from build123d import *

# Parameters (mm, degrees)
CROQUIS1_R              = 7.5
SALIENTE_EXTRUIR2_DEPTH = 30
REDONDEO1_R             = 25
CROQUIS2_R              = 7.5
SALIENTE_EXTRUIR3_DEPTH = 50
REDONDEO2_R             = 5
REDONDEO4_R             = 15


# Some blends are built 0.0001 mm under size
with BuildPart() as part:
    # Croquis1 → Saliente-Extruir2 (new body)
    with BuildSketch(Plane.XY):
        Polygon((12.5, 0), (12.5, 60), (37.5, 60), (37.5, 0), (50, 0), (50, 350), (0, 350), (0, 0), align=None)
        with Locations((25, 325)):
            Circle(CROQUIS1_R, mode=Mode.SUBTRACT)
    extrude(amount=SALIENTE_EXTRUIR2_DEPTH)

    # Redondeo1
    redondeo1_edges = [part.edges().sort_by_distance(p)[0] for p in [
        (0, 350, 15),
        (50, 350, 15),
    ]]
    fillet(redondeo1_edges, radius=REDONDEO1_R - 0.0001)  # a hair under: the kernel refuses the full size

    # Croquis2 → Saliente-Extruir3 (add)
    with BuildSketch(Plane.ZY):
        with Locations((15, 25)):
            Circle(CROQUIS2_R)
    extrude(amount=-SALIENTE_EXTRUIR3_DEPTH)

    # Redondeo2
    redondeo2_edges = [part.edges().sort_by_distance(p)[0] for p in [
        (12.5, 30, 30),
        (25, 60, 30),
        (50, 0, 15),
        (37.5, 0, 15),
        (12.5, 0, 15),
        (0, 0, 15),
        (37.5, 30, 30),
        (50, 162.50005, 30),
        (0, 162.50005, 0),
        (0, 162.50005, 30),
        (42.677698819, 342.677698819, 0),
        (7.322301181, 342.677698819, 0),
        (42.677698819, 342.677698819, 30),
        (7.322301181, 342.677698819, 30),
        (50, 162.50005, 0),
        (37.5, 30, 0),
        (25, 60, 0),
        (12.5, 30, 0),
    ]]
    fillet(redondeo2_edges, radius=REDONDEO2_R)

    # Redondeo4
    # the kernel refuses this fillet: 15 mm, written as the material it takes off along each edge
    with BuildSketch(Plane(origin=(50, 15, 15), x_dir=(0, -1, 0), z_dir=(0, 0, 1))) as redondeo4_piece_1:
        with BuildLine():
            CenterArc((10, -5), 5, 0, 90)
            Line((15, -5), (15, 0))
            Line((15, 0), (10, 0))
        make_face()
    revolve(axis=Axis((50, 15, 15), (1, 0, 0)), revolution_arc=90, mode=Mode.SUBTRACT)
    with BuildSketch(Plane(origin=(37.5, 15, 15), x_dir=(0, 0, -1), z_dir=(0, 1, 0))) as redondeo4_piece_2:
        with BuildLine():
            CenterArc((10, -5), 5, 0, 90)
            Line((15, -5), (15, 0))
            Line((15, 0), (10, 0))
        make_face()
    revolve(axis=Axis((37.5, 15, 15), (-1, 0, 0)), revolution_arc=90, mode=Mode.SUBTRACT)
    with BuildSketch(Plane(origin=(12.5, 15, 15), x_dir=(0, -1, 0), z_dir=(0, 0, 1))) as redondeo4_piece_3:
        with BuildLine():
            CenterArc((10, -5), 5, 0, 90)
            Line((15, -5), (15, 0))
            Line((15, 0), (10, 0))
        make_face()
    revolve(axis=Axis((12.5, 15, 15), (1, 0, 0)), revolution_arc=90, mode=Mode.SUBTRACT)
    with BuildSketch(Plane(origin=(0, 15, 15), x_dir=(0, 0, -1), z_dir=(0, 1, 0))) as redondeo4_piece_4:
        with BuildLine():
            CenterArc((10, -5), 5, 0, 90)
            Line((15, -5), (15, 0))
            Line((15, 0), (10, 0))
        make_face()
    revolve(axis=Axis((0, 15, 15), (-1, 0, 0)), revolution_arc=90, mode=Mode.SUBTRACT)
    with BuildSketch(Plane(origin=(12.5, 15, 15), x_dir=(0, 0, 1), z_dir=(0, 1, 0))) as redondeo4_piece_5:
        with BuildLine():
            CenterArc((10, -5), 5, 0, 90)
            Line((15, -5), (15, 0))
            Line((15, 0), (10, 0))
        make_face()
    revolve(axis=Axis((12.5, 15, 15), (1, 0, 0)), revolution_arc=90, mode=Mode.SUBTRACT)
    with BuildSketch(Plane(origin=(0, 15, 15), x_dir=(0, -1, 0), z_dir=(0, 0, -1))) as redondeo4_piece_6:
        with BuildLine():
            CenterArc((10, -5), 5, 0, 90)
            Line((15, -5), (15, 0))
            Line((15, 0), (10, 0))
        make_face()
    revolve(axis=Axis((0, 15, 15), (-1, 0, 0)), revolution_arc=90, mode=Mode.SUBTRACT)
    with BuildSketch(Plane(origin=(50, 15, 15), x_dir=(0, 0, 1), z_dir=(0, 1, 0))) as redondeo4_piece_7:
        with BuildLine():
            CenterArc((10, -5), 5, 0, 90)
            Line((15, -5), (15, 0))
            Line((15, 0), (10, 0))
        make_face()
    revolve(axis=Axis((50, 15, 15), (1, 0, 0)), revolution_arc=90, mode=Mode.SUBTRACT)
    with BuildSketch(Plane(origin=(37.5, 15, 15), x_dir=(0, -1, 0), z_dir=(0, 0, -1))) as redondeo4_piece_8:
        with BuildLine():
            CenterArc((10, -5), 5, 0, 90)
            Line((15, -5), (15, 0))
            Line((15, 0), (10, 0))
        make_face()
    revolve(axis=Axis((37.5, 15, 15), (-1, 0, 0)), revolution_arc=90, mode=Mode.SUBTRACT)
    with BuildSketch(Plane(origin=(37.5, 0, 30), x_dir=(0, 1, 0), z_dir=(1, 0, 0)), Plane(origin=(0, 0, 30), x_dir=(0, 1, 0), z_dir=(1, 0, 0))) as redondeo4_piece_9:
        with BuildLine():
            CenterArc((REDONDEO4_R, -REDONDEO4_R), REDONDEO4_R, 90, 90)
            Line((0, -REDONDEO4_R), (0, 0))
            Line((0, 0), (REDONDEO4_R, 0))
        make_face()
    extrude(amount=12.5, mode=Mode.SUBTRACT)
    with BuildSketch(Plane(origin=(0, 0, 0), x_dir=(0, 1, 0), z_dir=(1, 0, 0)), Plane(origin=(37.5, 0, 0), x_dir=(0, 1, 0), z_dir=(1, 0, 0))) as redondeo4_piece_10:
        with BuildLine():
            CenterArc((REDONDEO4_R, REDONDEO4_R), REDONDEO4_R, 180, 90)
            Line((0, REDONDEO4_R), (0, 0))
            Line((0, 0), (REDONDEO4_R, 0))
        make_face()
    extrude(amount=12.5, mode=Mode.SUBTRACT)


solid = part.part
Model file for the job. Use its own axes, mm. A direction names the side the tool comes from. Round coordinates to 2 decimals unless told otherwise and drop trailing zeros. Loops run counter-clockwise (first coordinate to the right, second up) from the corner with the lowest first, then second, coordinate; pieces in that order, holes last. Notation, with made-up numbers: (-20.75, 64) - (14.25, 64) arc R30 cw to (14.25, 100) - close; hole circle Ø1 at (-2.5, 47.25). An arc over 180 degrees is marked (long way). Write each question's results on one line, items separated by ' | '.
(1) 3-axis set-ups, long thin cutter, end or side, ignore diameter. For faces 4 (the flat face through (25, 60, 15)), 5 (the cylindrical face through (24.825, 32.436, 14.024)), 6 (the flat face through (50, 163, 15)): which of +Z, -Z, +X, -X, +Y, -Y reach the whole face in a straight line?
Answer below:
face 4: +Z, -Z | face 5: none | face 6: +Z, -Z, +X, +Y, -Y
(2) Saw through at A-A, the plane z = 15. Count the separate pieces of the cut face and the enclosed holes in it, then the cut area to 3 significant figures.
Answer below:
separate pieces: 1 | enclosed holes: 2 | area: 15,900 mm^2
(3) Wall check: L1, parallel to Y at x = 24.5, z = 15.25 (3 decimals); L2, parallel to Y at x = 25, z = 11; L3, parallel to X at y = 325, z = 19.25. Give the ranges that are in metal, low to high.
Answer below:
L1: y = 17.504 to 32.496, 60 to 317.517, 332.483 to 349.995 | L2: y = 18.66 to 31.34, 60 to 317.5, 332.5 to 350 | L3: x = 0 to 17.5, 32.5 to 50
(4) Pin check, flat tips, straight feed: pin 1 (10 mm diameter, centred on x = 30.5, z = 18, fed in from -Y); pin 2 (5 mm diameter, centred on x = 31, z = 21, fed in from -Y); pin 3 (1.5 mm diameter, centred on x = 26.5, z = 15, fed in from +Y). Stop position of each tip, or through.
Answer below:
pin 1: stops at y = 17.5 | pin 2: stops at y = 18.37 | pin 3: stops at y = 349.99
(5) Saw through at B-B, the plane y = 25. List the corners of the cut face in (x, z), then the cut area to 3 significant figures.
Answer below:
outline: (0, 5) arc R5 ccw to (5, 0) - (7.5, 0) arc R5 ccw to (12.5, 5) - (12.5, 7.5) - (37.5, 7.5) - (37.5, 5) arc R5 ccw to (42.5, 0) - (45, 0) arc R5 ccw to (50, 5) - (50, 25) arc R5 ccw to (45, 30) - (42.5, 30) arc R5 ccw to (37.5, 25) - (37.5, 22.5) - (12.5, 22.5) - (12.5, 25) arc R5 ccw to (7.5, 30) - (5, 30) arc R5 ccw to (0, 25) - close | area: 1,080 mm^2
(6) Mould opens along X. For faces 1 (the cylindrical face through (6, 0, 15)), 2 (the flat face through (37.5, 33, 15)), 3 (the flat face through (0, 167, 15)) say: released by +X, released by -X, zero draft, split by the parting line, or undercut.
Answer below:
face 1: zero draft | face 2: undercut | face 3: released by -X
